Read the model definition and answer for the solid it produces. Units are mm, in the model's axes. Face numbers are marked on the shaded views. A direction names the side the tool comes from. Give positions to 0.01 mm unless a question says otherwise; leave off trailing zeros. Loops run counter-clockwise (first coordinate to the right, second up) from the corner with the lowest first, then second, coordinate; pieces in that order, holes last. Notation, with made-up numbers: (82, 49) - (103, 49) arc R25 cw to (103, 61) - close; hole circle Ø5 at (76, -12). An arc over 180 degrees is marked (long way). Write each question's results on one line, items separated by ' | '. Start each with the question number.
Q1. The part is cut by section C-C, the plane z = 0. Write down the section's boundary in (x, y), plus the area to 3 significant figures.
Q2. The part is cut by section D-D, the plane y = 7.25. Write down the section's boundary in (x, z), plus the area to 3 significant figures.
Q3. Given pin 1 (5 mm diameter, centred on y = -1.5, z = 1.5, fed in from -X); pin 2 (8 mm diameter, centred on x = -24, z = 0, fed in from -Y); pin 3 (3 mm diameter, centred on y = 2.5, z = -4, fed in from +X); pin 4 (5.5 mm diameter, centred on x = 0, z = 24.46, fed in from -Y), each flat-ended and moving along its own axis, determine where each tip first touches the part or whether it passes through.
Q4. For the marked faces 1, 2, 3 and 4, determine the directions among +Z, -Z, +X, -X, +Y, -Y from which every point of the face is accessible in a straight line to the end or side of a thin tool.
Q5. The part is cut by section A-A, the plane x = 24. Write down the section's boundary in (y, z).
Q6. Find the intervals of material crossed by line 1 (Z direction, x = 0, y = 7.25); line 2 (Y direction, x = 6.5, z = -25.5); line 3 (X direction, y = -4, z = -36), in increasing order. Write a range as from..to.
Q7. The part is cut by section B-B, the plane z = 25. Write down the section's boundary in (x, y), plus the area to 3 significant figures.
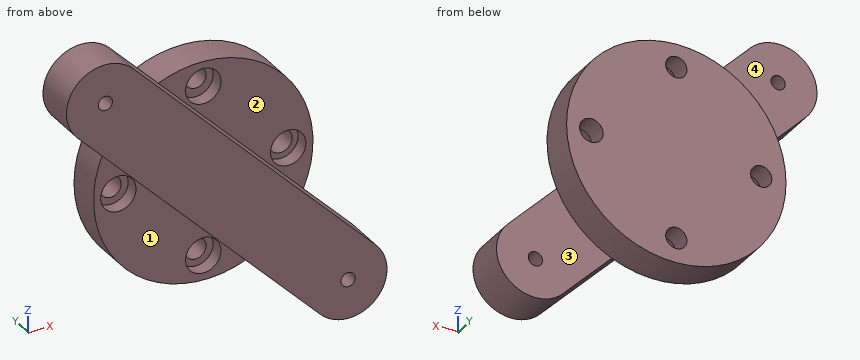
```python
from build123d import *

# Parameters (mm, degrees)
SKETCH1_R           = 31
BOSS_EXTRUDE1_DEPTH = 10
SKETCH3_R           = 5
CUT_EXTRUDE1_DEPTH  = 4
SKETCH5_R           = 5
CUT_EXTRUDE2_DEPTH  = 4
SKETCH6_R           = 3
SKETCH6_R_2         = 3.329647993
CUT_EXTRUDE3_DEPTH  = 10
SKETCH10_R          = 2
BOSS_EXTRUDE5_DEPTH = 12


with BuildPart() as part:
    # Sketch1 → Boss-Extrude1 (new body)
    with BuildSketch(Plane(origin=(0, 0, 0), x_dir=(1, 0, 0), z_dir=(0, 1, 0))):
        with Locations(Location((0, 0, 0), (0, 0, 270))):
            Circle(SKETCH1_R)
    extrude(amount=BOSS_EXTRUDE1_DEPTH)

    # Sketch3 → Cut-Extrude1 (cut)
    with BuildSketch(Plane(origin=(0, 0, 0), x_dir=(1, 0, 0), z_dir=(0, 1, 0))):
        with Locations(Location((0, 24, 0), (0, 0, 270))):
            Circle(SKETCH3_R)
    extrude(amount=CUT_EXTRUDE1_DEPTH, mode=Mode.SUBTRACT)

    # Sketch5 → Cut-Extrude2 (cut)
    with BuildSketch(Plane(origin=(0, 0, 0), x_dir=(1, 0, 0), z_dir=(0, 1, 0))):
        with Locations(Location((-24, 0, 0), (0, 0, 270))):
            Circle(SKETCH5_R)
        with Locations(Location((24, 0, 0), (0, 0, 270))):
            Circle(SKETCH5_R)
        with Locations(Location((0, -24, 0), (0, 0, 270))):
            Circle(SKETCH5_R)
    extrude(amount=CUT_EXTRUDE2_DEPTH, mode=Mode.SUBTRACT)

    # Sketch6 → Cut-Extrude3 (cut)
    with BuildSketch(Plane(origin=(0, 0, 0), x_dir=(1, 0, 0), z_dir=(0, 1, 0))):
        with Locations(Location((0, -24.460265292, 0), (0, 0, 270))):
            Circle(SKETCH6_R)
        with Locations(Location((-24, 0, 0), (0, 0, 270))):
            Circle(SKETCH6_R)
        with Locations(Location((24, 0, 0), (0, 0, 270))):
            Circle(SKETCH6_R_2)
        with Locations(Location((0, 24, 0), (0, 0, 270))):
            Circle(SKETCH6_R)
    extrude(amount=CUT_EXTRUDE3_DEPTH, mode=Mode.SUBTRACT)

    # Sketch10 → Boss-Extrude5 (add)
    with BuildSketch(Plane(origin=(0, 0, 0), x_dir=(1, 0, 0), z_dir=(0, 1, 0))):
        with BuildLine():
            Line((-42.072853481, -26.516504294), (26.516504294, 42.072853481))
            ThreePointArc((26.516504294, 42.072853481), (42.072853481, 42.072853481), (42.072853481, 26.516504294))
            Line((42.072853481, 26.516504294), (-26.516504294, -42.072853481))
            ThreePointArc((-26.516504294, -42.072853481), (-42.072853481, -42.072853481), (-42.072853481, -26.516504294))
        make_face()
        with Locations(Location((34.294678888, 34.294678888, 0), (0, 0, 270))):
            Circle(SKETCH10_R, mode=Mode.SUBTRACT)
        with Locations(Location((-34.294678888, -34.294678888, 0), (0, 0, 270))):
            Circle(SKETCH10_R, mode=Mode.SUBTRACT)
    extrude(amount=-BOSS_EXTRUDE5_DEPTH)


solid = part.part
```
Check sheet entries:
1) outline: (-31, 0) - (-29, 0) - (-29, 4) - (-27, 4) - (-27, 10) - (-31, 10) - close; (-21, 4) - (-19, 4) - (-19, 0) - (-15.56, 0) - (-15.56, -12) - (15.56, -12) - (15.56, 0) - (19, 0) - (19, 4) - (20.67, 4) - (20.67, 10) - (-21, 10) - close; (27.33, 4) - (29, 4) - (29, 0) - (31, 0) - (31, 10) - (27.33, 10) - close | area: 837 mm^2
2) outline: circle Ø62 at (0, 0); hole circle Ø6 at (-24, 0); hole circle Ø6 at (0, -24); hole circle Ø6 at (0, 24.46); hole circle Ø6.66 at (24, 0) | area: 2,900 mm^2
3) pin 1: stops at x = -31 | pin 2: stops at y = 4 | pin 3: stops at x = 30.9 | pin 4: passes through
4) face 1: -Z, -X, -Y | face 2: +Z, +X, -Y | face 3: -Z, +X, +Y | face 4: +Z, -X, +Y
5) outline: (-12, -39.56) - (0, -39.56) - (0, -19.62) - (10, -19.62) - (10, -3.33) - (4, -3.33) - (4, -5) - (0, -5) - (0, -8.44) - (-12, -8.44) - close; (0, 5) - (4, 5) - (4, 3.33) - (10, 3.33) - (10, 19.62) - (0, 19.62) - close
6) line 1: z = -31..-27, -21..21.46, 27.46..31 | line 2: y = 0..10 | line 3: x = 20.44..33.25, 35.34..45.16
7) outline: (-40.56, -12) - (-9.44, -12) - (-9.44, 0) - (-4.9, 0) - (-4.9, 4) - (-2.95, 4) - (-2.95, 10) - (-18.33, 10) - (-18.33, 0) - (-40.56, 0) - close; (2.95, 4) - (4.9, 4) - (4.9, 0) - (18.33, 0) - (18.33, 10) - (2.95, 10) - close | area: 665 mm^2
